Geometry check sheet. Reference: the model listing, model coordinates, mm. Coordinates: 2 decimals unless noted, no trailing zeros. Write each loop counter-clockwise with the first axis right and the second up, starting at its lowest first coordinate (ties: lowest second). Pieces come first, ordered by that corner, then holes.
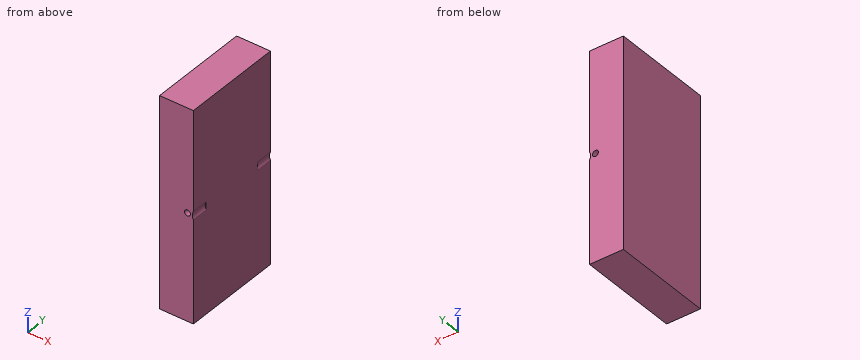
from build123d import *

# Parameters (mm, degrees)
SKETCH1_W           = 20
SKETCH1_H           = 60
BOSS_EXTRUDE1_DEPTH = 62
SKETCH2_R           = 5.1
CUT_EXTRUDE1_DEPTH  = 10
SKETCH3_R           = 4
SKETCH3_R_2         = 1.75
CUT_EXTRUDE2_DEPTH  = 87.856203002


with BuildPart() as part:
    # Sketch1 → Boss-Extrude1 (new, symmetric)
    with BuildSketch(Plane.XY):
        Rectangle(SKETCH1_W, SKETCH1_H)
    extrude(amount=BOSS_EXTRUDE1_DEPTH, both=True)

    # Sketch2 → Cut-Extrude1 (cut)
    with BuildSketch(Plane(origin=(0, 30, 0), x_dir=(1, 0, 0), z_dir=(0, 1, 0))):
        with Locations((14.5, -1)):
            Circle(SKETCH2_R)
    cut_extrude1 = extrude(amount=-CUT_EXTRUDE1_DEPTH, mode=Mode.SUBTRACT)

    # Mirror1: Cut-Extrude1 across plane
    add(cut_extrude1.mirror(Plane.ZX), mode=Mode.SUBTRACT)

    # Sketch3 → Cut-Extrude2 (cut, through all)
    with BuildSketch(Plane(origin=(0, 30, 0), x_dir=(1, 0, 0), z_dir=(0, 1, 0))):
        with Locations((14.5, -1)):
            Circle(SKETCH3_R)
        with Locations(Location((6.5, -1, 0), (0, 0, 270))):
            Circle(SKETCH3_R_2)
        with Locations((14.5, 7)):
            Circle(SKETCH3_R_2)
        with Locations((22.5, -1)):
            Circle(SKETCH3_R_2)
        with Locations((14.5, -9)):
            Circle(SKETCH3_R_2)
    extrude(amount=-CUT_EXTRUDE2_DEPTH, mode=Mode.SUBTRACT)


solid = part.part
1. Gauge pin test, flat end, axial feed: pin 1 Ø0.5 at (x, z) = (10, 1.5) entering from +Y. Record the tip position at first contact, or that the pin passes through.
Computed values:
pin 1: stops at y = 20
2. Sectioned sample at B-B, the plane x = 6.5. Record the boundary of the cut face in (y, z).
Computed values:
outline: (-30, -62) - (30, -62) - (30, -0.75) - (-30, -0.75) - close; (-30, 2.75) - (30, 2.75) - (30, 62) - (-30, 62) - close
3. Thickness scan on line 1 along X through (y, z) = (-4, 1); line 2 along X through (y, z) = (-23, 2); line 3 along Z through (x, y) = (7.5, 16.5). Record the ranges inside material, lowest first.
Computed values:
line 1: x = -10 to 4.75, 8.25 to 10
line 2: x = -10 to 5.06, 7.94 to 9.5
line 3: z = -62 to -0.44, 2.44 to 62
4. Sectioned sample at A-A, the plane z = 1. Record the boundary of the cut face in (x, y), and give its area (3 significant figures).
Computed values:
outline: (-10, -30) - (4.75, -30) - (4.75, 30) - (-10, 30) - close; (8.25, -30) - (9.4, -30) - (9.4, -20) - (10, -20) - (10, 20) - (9.4, 20) - (9.4, 30) - (8.25, 30) - close
area: 978 mm2
